```python
from build123d import *

# Parameters (mm, degrees)
F4_T = -2.5


with BuildPart() as f3:
    # F0 (on Top) → F3 section 0
    with BuildSketch(Plane.XY):
        with BuildLine():
            Line((25, 30), (-25, 30))
            ThreePointArc((-25, 30), (-28.5355339059, 28.5355339059), (-30, 25))
            Line((-30, 25), (-30, -25))
            ThreePointArc((-30, -25), (-28.5355339059, -28.5355339059), (-25, -30))
            Line((-25, -30), (25, -30))
            ThreePointArc((25, -30), (28.5355339059, -28.5355339059), (30, -25))
            Line((30, -25), (30, 25))
            ThreePointArc((30, 25), (28.5355339059, 28.5355339059), (25, 30))
        make_face()
    # F2 (on offset) → F3 section 1
    with BuildSketch(Plane.XY.offset(45)):
        with BuildLine():
            Line((52.5, 62.5), (-52.5, 62.5))
            ThreePointArc((-52.5, 62.5), (-59.5710678119, 59.5710678119), (-62.5, 52.5))
            Line((-62.5, 52.5), (-62.5, -52.5))
            ThreePointArc((-62.5, -52.5), (-59.5710678119, -59.5710678119), (-52.5, -62.5))
            Line((-52.5, -62.5), (52.5, -62.5))
            ThreePointArc((52.5, -62.5), (59.5710678119, -59.5710678119), (62.5, -52.5))
            Line((62.5, -52.5), (62.5, 52.5))
            ThreePointArc((62.5, 52.5), (59.5710678119, 59.5710678119), (52.5, 62.5))
        make_face()
    loft()

    # F4
    f4_openings = [f3.faces().sort_by_distance(p)[0] for p in [
        (0, 0, 45),
    ]]
    offset(amount=F4_T, openings=f4_openings)


solid = f3.part
```
Can you work these out from the model? Positions are in its coordinate system, mm. A direction names the side the tool comes from. Coordinates: 2 decimals unless noted, no trailing zeros.
Item 1: If we mould it in two halves opening along X, with no side actions, what happens to faces 1 (the face through (0, 0, 0)), 2 (the face through (0.722, 47.694, 28.77))? For each: released by +X, released by -X, zero draft, split by the parting line, or undercut.
Answers below:
face 1: zero draft
face 2: undercut
Item 2: I'm going to push flat-ended pins straight in: pin 1 (12 mm diameter, centred on x = -34.5, z = 8, fed in from -Y); pin 2 (5 mm diameter, centred on y = -33, z = 20, fed in from +X); pin 3 (3 mm diameter, centred on x = -40, z = 33, fed in from -Y); pin 4 (6 mm diameter, centred on y = -46, z = 12, fed in from -X). Where does each tip first touch, or does it pass through?
Answers below:
pin 1: stops at y = -40.08
pin 2: stops at x = 46.25
pin 3: stops at y = -54.92
pin 4: passes through
Item 3: Please list where these lines run through material, in increasing order: L1, parallel to Z at x = 17.5, y = -12; L2, parallel to X at y = -20.5, z = 18; L3, parallel to Y at x = 16.5, z = 11.
Answers below:
L1: z = 0 to 2.5
L2: x = -43 to -39.92, 39.92 to 43
L3: y = -37.94 to -34.86, 34.86 to 37.94
Item 4: Which directions (+Z, -Z, +X, -X, +Y, -Y) give clear straight access to the entire face, cutting with the end or side of a thin tool? Please do faces 3 (the face through (-60, 0, 45)), 4 (the face through (0, 0, 2.5)).
Answers below:
face 3: +Z, +X, -X, +Y, -Y
face 4: +Z
